Verification items for the finished model (mm, model axes). A direction names the side the tool comes from. Round coordinates to 2 decimals unless told otherwise and drop trailing zeros. Order: outer loops, then holes, each group sorted by start corner. A loop starts at its lowest first (then second) coordinate and runs counter-clockwise, first axis right, second up. Notation, with made-up numbers: (48, -20.75) -> (95, -20.75) arc R17 ccw to (95, 9.25) -> close; hole circle Ø5 at (-23, 70). An arc over 180 degrees is marked (long way). Put each result on its own line as item: value.
```python
from build123d import *

# Parameters (mm, degrees)
ESBO_O1_R                = 12.5
RESSALTO_EXTRUS_O1_DEPTH = 20.8
ESBO_O2_R                = 12.1
RESSALTO_EXTRUS_O2_DEPTH = 29.8
ESBO_O3_R                = 2
RESSALTO_EXTRUS_O3_DEPTH = 11.8
CORTE_EXTRUS_O1_START    = -8.1
CORTE_EXTRUS_O1_DEPTH    = 8.1
ESBO_O5_R                = 3.5
RESSALTO_EXTRUS_O4_DEPTH = 2
ESBO_O6_R                = 1.5
CORTE_EXTRUS_O2_DEPTH    = 10
RESSALTO_EXTRUS_O5_START = 9
ESBO_O8_R                = 1.5
RESSALTO_EXTRUS_O5_DEPTH = 9
CORTE_EXTRUS_O3_DEPTH    = 0.5
ESBO_O10_R               = 4.25
RESSALTO_EXTRUS_O6_DEPTH = 2.8
ESBO_O11_W               = 2
ESBO_O11_H               = 0.4
RESSALTO_EXTRUS_O8_DEPTH = 6
FILETE1_R                = 1
CORTE_EXTRUS_O4_DEPTH    = 22


with BuildPart() as part:
    # Esboço1 → Ressalto-extrusão1 (new body)
    with BuildSketch(Plane(origin=(0, 0, 0), x_dir=(1, 0, 0), z_dir=(0, 1, 0))):
        with Locations(Location((0, 0, 0), (0, 0, 270))):
            Circle(ESBO_O1_R)
    extrude(amount=RESSALTO_EXTRUS_O1_DEPTH)

    # Esboço2 → Ressalto-extrusão2 (add)
    with BuildSketch(Plane(origin=(0, 0, 0), x_dir=(-1, 0, 0), z_dir=(0, -1, 0))):
        with Locations(Location((0, 0, 0), (0, 0, 90))):
            Circle(ESBO_O2_R)
    extrude(amount=RESSALTO_EXTRUS_O2_DEPTH)

    # Esboço3 → Ressalto-extrusão3 (add)
    with BuildSketch(Plane(origin=(0, 20.8, 0), x_dir=(1, 0, 0), z_dir=(0, 1, 0))):
        with Locations(Location((0, 0, 0), (0, 0, 270))):
            Circle(ESBO_O3_R)
    extrude(amount=RESSALTO_EXTRUS_O3_DEPTH)

    # Esboço4 → Corte-extrusão1 (cut)
    with BuildSketch(Plane(origin=(0, 32.6, 0), x_dir=(1, 0, 0), z_dir=(0, 1, 0)).offset(CORTE_EXTRUS_O1_START)):
        with BuildLine():
            Line((-1.702650866, 1.049275955), (1.702650866, 1.049275955))
            ThreePointArc((1.702650866, 1.049275955), (0, 2), (-1.702650866, 1.049275955))
        make_face()
    extrude(amount=CORTE_EXTRUS_O1_DEPTH, mode=Mode.SUBTRACT)

    # Esboço5 → Ressalto-extrusão4 (add)
    with BuildSketch(Plane(origin=(0, 20.8, 0), x_dir=(1, 0, 0), z_dir=(0, 1, 0))):
        with Locations(Location((0, 0, 0), (0, 0, 270))):
            Circle(ESBO_O5_R)
    extrude(amount=RESSALTO_EXTRUS_O4_DEPTH)

    # Esboço6 → Corte-extrusão2 (cut)
    with BuildSketch(Plane(origin=(0, 20.8, 0), x_dir=(1, 0, 0), z_dir=(0, 1, 0))):
        with Locations(Location((0, 8.5, 0), (0, 0, 270))):
            Circle(ESBO_O6_R)
        with Locations(Location((8.5, 0, 0), (0, 0, 270))):
            Circle(ESBO_O6_R)
        with Locations(Location((0, -8.5, 0), (0, 0, 270))):
            Circle(ESBO_O6_R)
        with Locations(Location((-8.5, 0, 0), (0, 0, 270))):
            Circle(ESBO_O6_R)
    extrude(amount=-CORTE_EXTRUS_O2_DEPTH, mode=Mode.SUBTRACT)

    # Esboço8 → Ressalto-extrusão5 (add)
    with BuildSketch(Plane(origin=(0, 10.8, 0), x_dir=(1, 0, 0), z_dir=(0, 1, 0)).offset(RESSALTO_EXTRUS_O5_START)):
        with Locations(Location((0, 8.5, 0), (0, 0, 270))):
            Circle(ESBO_O8_R)
        with Locations(Location((0, -8.5, 0), (0, 0, 270))):
            Circle(ESBO_O8_R)
    extrude(amount=-RESSALTO_EXTRUS_O5_DEPTH)

    # Esboço9 → Corte-extrusão3 (cut)
    with BuildSketch(Plane(origin=(0, 19.8, 0), x_dir=(1, 0, 0), z_dir=(0, 1, 0))):
        with BuildLine():
            Line((-0.3, 8.2), (-0.3, 7.75))
            ThreePointArc((-0.3, 7.75), (0, 7.45), (0.3, 7.75))
            Line((0.3, 7.75), (0.3, 8.2))
            Line((0.3, 8.2), (0.75, 8.2))
            ThreePointArc((0.75, 8.2), (1.05, 8.5), (0.75, 8.8))
            Line((0.75, 8.8), (0.3, 8.8))
            Line((0.3, 8.8), (0.3, 9.25))
            ThreePointArc((0.3, 9.25), (0, 9.55), (-0.3, 9.25))
            Line((-0.3, 9.25), (-0.3, 8.8))
            Line((-0.3, 8.8), (-0.75, 8.8))
            ThreePointArc((-0.75, 8.8), (-1.05, 8.5), (-0.75, 8.2))
            Line((-0.75, 8.2), (-0.3, 8.2))
        make_face()
        with BuildLine():
            Line((0.3, -8.2), (0.3, -7.75))
            ThreePointArc((0.3, -7.75), (0, -7.45), (-0.3, -7.75))
            Line((-0.3, -7.75), (-0.3, -8.2))
            Line((-0.3, -8.2), (-0.75, -8.2))
            ThreePointArc((-0.75, -8.2), (-1.05, -8.5), (-0.75, -8.8))
            Line((-0.75, -8.8), (-0.3, -8.8))
            Line((-0.3, -8.8), (-0.3, -9.25))
            ThreePointArc((-0.3, -9.25), (0, -9.55), (0.3, -9.25))
            Line((0.3, -9.25), (0.3, -8.8))
            Line((0.3, -8.8), (0.75, -8.8))
            ThreePointArc((0.75, -8.8), (1.05, -8.5), (0.75, -8.2))
            Line((0.75, -8.2), (0.3, -8.2))
        make_face()
    extrude(amount=-CORTE_EXTRUS_O3_DEPTH, mode=Mode.SUBTRACT)

    # Esboço10 → Ressalto-extrusão6 (add)
    with BuildSketch(Plane.XZ.offset(29.8)):
        with Locations(Location((0, 0, 0), (0, 0, 270))):
            Circle(ESBO_O10_R)
    extrude(amount=RESSALTO_EXTRUS_O6_DEPTH)

    # Esboço11 → Ressalto-extrusão8 (add)
    with BuildSketch(Plane(origin=(0, -29.8, 0), x_dir=(-1, 0, 0), z_dir=(0, -1, 0))):
        with Locations((0, 8.9)):
            Rectangle(ESBO_O11_W, ESBO_O11_H)
        with Locations((0, -8.9)):
            Rectangle(ESBO_O11_W, ESBO_O11_H)
    extrude(amount=RESSALTO_EXTRUS_O8_DEPTH)

    # Filete1
    filete1_edges = [part.edges().sort_by_distance(p)[0] for p in [
        (1, -35.8, -8.9),
        (-1, -35.8, -8.9),
        (-1, -35.8, 8.9),
        (1, -35.8, 8.9),
    ]]
    fillet(filete1_edges, radius=FILETE1_R - 0.0001)  # a hair under: the kernel refuses the full size

    # Esboço12 → Corte-extrusão4 (cut)
    with BuildSketch(Plane.XY.offset(9.1)):
        with BuildLine():
            Line((0.355764182, -33.51076438), (0.355764182, -34.668869147))
            ThreePointArc((0.355764182, -34.668869147), (0, -35.024633329), (-0.355764182, -34.668869147))
            Line((-0.355764182, -34.668869147), (-0.355764182, -33.51076438))
            ThreePointArc((-0.355764182, -33.51076438), (0, -33.155000198), (0.355764182, -33.51076438))
        make_face()
    extrude(amount=-CORTE_EXTRUS_O4_DEPTH, mode=Mode.SUBTRACT)


solid = part.part
```
Item 1: Sectioned sample at C-C, the plane x = 2.75. Record the boundary of the cut face in (y, z), then the cut area to 3 significant figures.
Geometry check:
outline: (-32.6, -3.24) -> (-29.8, -3.24) -> (-29.8, -11.78) -> (0, -11.78) -> (0, -12.19) -> (20.8, -12.19) -> (20.8, -2.17) -> (22.8, -2.17) -> (22.8, 2.17) -> (20.8, 2.17) -> (20.8, 12.19) -> (0, 12.19) -> (0, 11.78) -> (-29.8, 11.78) -> (-29.8, 3.24) -> (-32.6, 3.24) -> close
area: 1,240 mm2
Item 2: Release check for a two-part mould opening along X. For faces 5 (the face through (0, 19.3, 8)), 6 (the face through (0, -29.8, -5)), 7 (the face through (-0.766, 27.631, 1.847)), 8 (the face through (0, 19.3, -9)) record: pulls with the +X half, pulls with the -X half, needs draft (parallel to the pull), parting line crosses it, or undercut.
Geometry check:
face 5: undercut
face 6: needs draft
face 7: parting line crosses it
face 8: undercut
Item 3: Sectioned sample at B-B, the plane y = 17. Record the boundary of the cut face in (x, z), then the cut area to 3 significant figures.
Geometry check:
outline: circle Ø25 at (0, 0); hole circle Ø3 at (-8.5, 0); hole circle Ø3 at (8.5, 0)
area: 477 mm2
Item 4: Sectioned sample at D-D, the plane y = -24. Record the boundary of the cut face in (x, z), then the cut area to 3 significant figures.
Geometry check:
outline: circle Ø24.2 at (0, 0)
area: 460 mm2
Item 5: Material ranges on line 1 along X through (y, z) = (16, 0); line 2 along Y through (x, z) = (-8, 9); line 3 along Z through (x, y) = (0.5, 15.5), recorded low to high.
Geometry check:
line 1: -12.5 to -10, -7 to 7, 10 to 12.5
line 2: -29.8 to 20.8
line 3: -12.49 to 12.49
Item 6: Tool access check on faces 1 (the face through (0, -33, -9.1)), 2 (the face through (7, 16, 0)), 3 (the face through (0, -32.6, 0)), 4 (the face through (4.214, -31.18, 0.553)). Record the directions out of +Z, -Z, +X, -X, +Y, -Y that give a thin tool (end or side, any length) a straight path to the whole face; none if there is none.
Geometry check:
face 1: -Z, +X, -X, -Y
face 2: +Y
face 3: +X, -X, -Y
face 4: -Y
Item 7: Sectioned sample at A-A, the plane y = -31. Record the boundary of the cut face in (x, z).
Geometry check:
outline: circle Ø8.5 at (0, 0); (-1, -9.1) -> (1, -9.1) -> (1, -8.7) -> (-1, -8.7) -> close; (-1, 8.7) -> (1, 8.7) -> (1, 9.1) -> (-1, 9.1) -> close
Item 8: Depth check by flat-ended pin: pin 1 Ø3.5 at (x, z) = (0, 8.5) entering from +Y; pin 2 Ø10 at (x, z) = (-6, 8) entering from -Y; pin 3 Ø1.5 at (x, z) = (0, -8) entering from +Y. Enter the tip coordinate at first touch or a pass-through.
Geometry check:
pin 1: y = 20.8
pin 2: y = -29.8
pin 3: y = 19.8
